Here's how the part is built. I have some questions about the finished solid (model axes, mm). Face numbers are marked on the shaded views. Coordinates: 2 decimals unless noted, no trailing zeros. Write each loop counter-clockwise with the first axis right and the second up, starting at its lowest first coordinate (ties: lowest second). Pieces come first, ordered by that corner, then holes. Notation, with made-up numbers: (66, 87) -> (100, 87) arc R20 ccw to (100, 108) -> close; hole circle Ø5 at (-21, 48.25). An arc over 180 degrees is marked (long way). Use a Markdown table: item, result. Add a question column.
Item 1: Imagine slicing it at C-C, the plane y = 48.25. Write out the boundary of the cut face in (x, z), and give its area (3 significant figures).
Item 2: Imagine slicing it at B-B, the plane x = -5.08. Write out the boundary of the cut face in (y, z), and give its area (3 significant figures).
Item 3: Imagine slicing it at A-A, the plane z = 46.99. Write out the boundary of the cut face in (x, y).
Item 4: If we mould it in two halves opening along Z, with no side actions, what happens to the marked faces 1, 2, 3 and 4? For each: pulls with the +Z half, pulls with the -Z half, needs draft (parallel to the pull), parting line crosses it, or undercut.
Item 5: If I drill on line 1 along Z through (x, y) = (-5.08, 43); line 2 along Z through (x, y) = (42, 47.25); line 3 along X through (y, z) = (44.25, 45.5), over which ranges is the centre line in solid material (lowest first)? Write a range as from..to.
```python
from build123d import *

# Parameters (mm, degrees)
BOSS_EXTRUDE1_DEPTH = 50.8
CUT_EXTRUDE1_REACH  = 70.151
SKETCH2_R           = 7.62
SKETCH3_R           = 2.1828125
CUT_EXTRUDE2_DEPTH  = 69.150694513


with BuildPart() as part:
    # Sketch1 → Boss-Extrude1 (new body)
    with BuildSketch(Plane.XY):
        Polygon((-8.89, 40.64), (-8.89, 46.99), (-8.89, 49.53), (44.5516, 49.53), (44.5516, 46.99), (44.5516, 40.64), align=None)
    extrude(amount=BOSS_EXTRUDE1_DEPTH)

    # Sketch2 → Cut-Extrude1 (cut, up to next)
    with BuildSketch(Plane(origin=(0, 49.53, 0), x_dir=(1, 0, 0), z_dir=(0, 1, 0)), mode=Mode.PRIVATE) as cut_extrude1_sk1:
        with Locations(Location((17.8798, -32.350999872, 0), (0, 0, 180))):
            Circle(SKETCH2_R)
    cut_extrude1_tool1 = extrude(cut_extrude1_sk1.sketch, amount=-CUT_EXTRUDE1_REACH, mode=Mode.PRIVATE) & part.part
    add(cut_extrude1_tool1.solids().sort_by_distance((17.8798, 49.53, 32.351))[0], mode=Mode.SUBTRACT)

    # Sketch3 → Cut-Extrude2 (cut, through all)
    with BuildSketch(Plane(origin=(0, 49.53, 0), x_dir=(1, 0, 0), z_dir=(0, 1, 0))):
        with Locations(Location((40.7416, -46.99, 0), (0, 0, 180))):
            Circle(SKETCH3_R)
        with Locations(Location((-5.08, -46.99, 0), (0, 0, 180))):
            Circle(SKETCH3_R)
        with Locations(Location((-5.08, -3.81, 0), (0, 0, 180))):
            Circle(SKETCH3_R)
        with Locations(Location((40.7416, -3.81, 0), (0, 0, 180))):
            Circle(SKETCH3_R)
    extrude(amount=-CUT_EXTRUDE2_DEPTH, mode=Mode.SUBTRACT)


solid = part.part
```
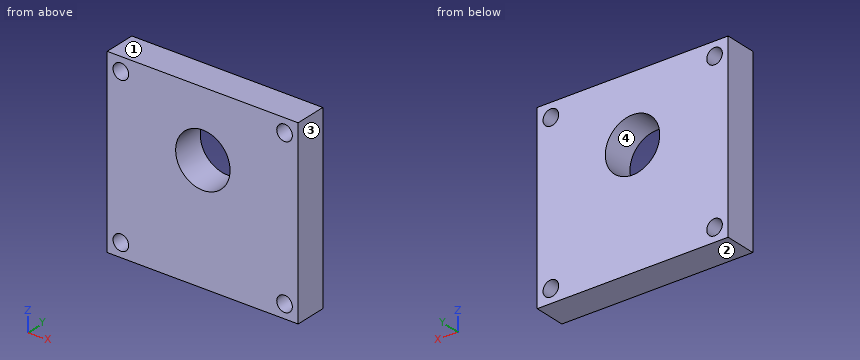
Ans:
| question | item | result |
|---|---|---|
| 1 | outline | (-8.89, 0) -> (44.55, 0) -> (44.55, 50.8) -> (-8.89, 50.8) -> close; hole circle Ø4.37 at (-5.08, 3.81); hole circle Ø4.37 at (-5.08, 46.99); hole circle Ø15.24 at (17.88, 32.35); hole circle Ø4.37 at (40.74, 3.81); hole circle Ø4.37 at (40.74, 46.99) |
| 1 | area | 2,470 mm^2 |
| 2 | outline | (40.64, 0) -> (49.53, 0) -> (49.53, 1.63) -> (40.64, 1.63) -> close; (40.64, 5.99) -> (49.53, 5.99) -> (49.53, 44.81) -> (40.64, 44.81) -> close; (40.64, 49.17) -> (49.53, 49.17) -> (49.53, 50.8) -> (40.64, 50.8) -> close |
| 2 | area | 374 mm^2 |
| 3 | outline | (-8.89, 40.64) -> (-7.26, 40.64) -> (-7.26, 49.53) -> (-8.89, 49.53) -> close; (-2.9, 40.64) -> (38.56, 40.64) -> (38.56, 49.53) -> (-2.9, 49.53) -> close; (42.92, 40.64) -> (44.55, 40.64) -> (44.55, 49.53) -> (42.92, 49.53) -> close |
| 4 | face 1 | pulls with the +Z half |
| 4 | face 2 | pulls with the -Z half |
| 4 | face 3 | needs draft |
| 4 | face 4 | undercut |
| 5 | line 1 | z = 0..1.63, 5.99..44.81, 49.17..50.8 |
| 5 | line 2 | z = 0..2.03, 5.59..45.21, 48.77..50.8 |
| 5 | line 3 | x = -8.89..-6.68, -3.48..39.15, 42.34..44.55 |
